CAD build for the part. Positions are in the model's coordinates, mm. Face numbers are marked on the shaded views. A direction names the side the tool comes from. Round coordinates to 2 decimals unless told otherwise and drop trailing zeros. Write each loop counter-clockwise with the first axis right and the second up, starting at its lowest first coordinate (ties: lowest second). Pieces come first, ordered by that corner, then holes. Notation, with made-up numbers: (65, 52.25) - (122, 52.25) arc R24 cw to (122, 62.25) - close; hole circle Ø3 at (35.5, -27.5). An arc over 180 degrees is marked (long way). Answer in a Markdown table with one row per item.
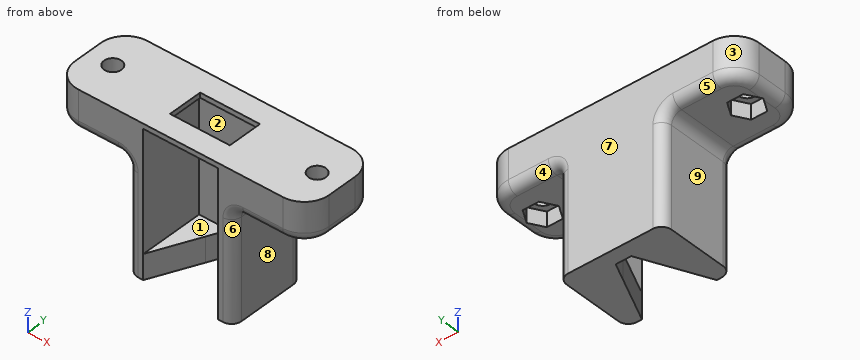
```python
from build123d import *

# Parameters (mm, degrees)
SKETCH1_W           = 15
SKETCH1_H           = 10
SKETCH1_W_2         = 12
SKETCH1_H_2         = 7
SKETCH1_H_3         = 3
SKETCH1_R           = 1.75
BOSS_EXTRUDE1_DEPTH = 1
BOSS_EXTRUDE2_DEPTH = 24
BOSS_EXTRUDE3_START = -7
SKETCH1_5_R         = 1.75
BOSS_EXTRUDE3_DEPTH = 7
BOSS_EXTRUDE4_DEPTH = 5
CUT_EXTRUDE1_DEPTH  = 20
FILLET1_R           = 2


with BuildPart() as part:
    # Sketch1 → Boss-Extrude1 (new body)
    # profile 1 of 7: a face of its own
    with BuildSketch(Plane.XY):
        with Locations((7.5, 5)):
            Rectangle(SKETCH1_W, SKETCH1_H)
        with Locations((7.5, 5)):
            Rectangle(SKETCH1_W_2, SKETCH1_H_2, mode=Mode.SUBTRACT)
    # profile 2 of 7: a face of its own
    with BuildSketch(Plane.XY):
        with Locations((7.5, -1.5)):
            Rectangle(SKETCH1_W, SKETCH1_H_3)
    # profile 3 of 7: a face of its own
    with BuildSketch(Plane.XY):
        Polygon((0, -3), (0, 0), (0, 10), (15, 10), (15, 0), (15, -3), (18, -3), (18, 13), (-3, 13), (-3, -3), align=None)
    # profile 4 of 7: a face of its own
    with BuildSketch(Plane.XY):
        with BuildLine():
            Line((-13, -3), (-3, -3))
            Line((-3, -3), (-3, 13))
            Line((-3, 13), (-13, 13))
            ThreePointArc((-13, 13), (-16.535533906, 11.535533906), (-18, 8))
            Line((-18, 8), (-18, 2))
            ThreePointArc((-18, 2), (-16.535533906, -1.535533906), (-13, -3))
        make_face()
        Polygon((-11.383419246, 7.8), (-9.766838493, 5), (-11.383419246, 2.2), (-14.616580754, 2.2), (-16.233161507, 5), (-14.616580754, 7.8), align=None, mode=Mode.SUBTRACT)
    # profile 5 of 7: a face of its own
    with BuildSketch(Plane.XY):
        Polygon((-14.616580754, 2.2), (-11.383419246, 2.2), (-9.766838493, 5), (-11.383419246, 7.8), (-14.616580754, 7.8), (-16.233161507, 5), align=None)
        with Locations((-13, 5)):
            Circle(SKETCH1_R, mode=Mode.SUBTRACT)
    # profile 6 of 7: a face of its own
    with BuildSketch(Plane.XY):
        with BuildLine():
            Line((18, 13), (18, -3))
            Line((18, -3), (28, -3))
            ThreePointArc((28, -3), (31.535533906, -1.535533906), (33, 2))
            Line((33, 2), (33, 8))
            ThreePointArc((33, 8), (31.535533906, 11.535533906), (28, 13))
            Line((28, 13), (18, 13))
        make_face()
        Polygon((26.383419246, 2.2), (24.766838493, 5), (26.383419246, 7.8), (29.616580754, 7.8), (31.233161507, 5), (29.616580754, 2.2), align=None, mode=Mode.SUBTRACT)
    # profile 7 of 7: a face of its own
    with BuildSketch(Plane.XY):
        Polygon((29.616580754, 7.8), (26.383419246, 7.8), (24.766838493, 5), (26.383419246, 2.2), (29.616580754, 2.2), (31.233161507, 5), align=None)
        with Locations((28, 5)):
            Circle(SKETCH1_R, mode=Mode.SUBTRACT)
    extrude(amount=BOSS_EXTRUDE1_DEPTH)

    # Sketch1<4> → Boss-Extrude2 (add)
    with BuildSketch(Plane.XY):
        Polygon((0, -3), (0, 0), (0, 10), (15, 10), (15, 0), (15, -3), (18, -3), (18, 13), (-3, 13), (-3, -3), align=None)
    extrude(amount=-BOSS_EXTRUDE2_DEPTH)

    # Sketch1<5> → Boss-Extrude3 (add)
    # profile 1 of 4: a face of its own
    with BuildSketch(Plane.XY.offset(BOSS_EXTRUDE3_START)):
        with BuildLine():
            Line((18, 13), (18, -3))
            Line((18, -3), (28, -3))
            ThreePointArc((28, -3), (31.535533906, -1.535533906), (33, 2))
            Line((33, 2), (33, 8))
            ThreePointArc((33, 8), (31.535533906, 11.535533906), (28, 13))
            Line((28, 13), (18, 13))
        make_face()
        Polygon((26.383419246, 2.2), (24.766838493, 5), (26.383419246, 7.8), (29.616580754, 7.8), (31.233161507, 5), (29.616580754, 2.2), align=None, mode=Mode.SUBTRACT)
    # profile 2 of 4: a face of its own
    with BuildSketch(Plane.XY.offset(BOSS_EXTRUDE3_START)):
        Polygon((29.616580754, 7.8), (26.383419246, 7.8), (24.766838493, 5), (26.383419246, 2.2), (29.616580754, 2.2), (31.233161507, 5), align=None)
        with Locations((28, 5)):
            Circle(SKETCH1_5_R, mode=Mode.SUBTRACT)
    # profile 3 of 4: a face of its own
    with BuildSketch(Plane.XY.offset(BOSS_EXTRUDE3_START)):
        with BuildLine():
            Line((-13, -3), (-3, -3))
            Line((-3, -3), (-3, 13))
            Line((-3, 13), (-13, 13))
            ThreePointArc((-13, 13), (-16.535533906, 11.535533906), (-18, 8))
            Line((-18, 8), (-18, 2))
            ThreePointArc((-18, 2), (-16.535533906, -1.535533906), (-13, -3))
        make_face()
        Polygon((-11.383419246, 7.8), (-9.766838493, 5), (-11.383419246, 2.2), (-14.616580754, 2.2), (-16.233161507, 5), (-14.616580754, 7.8), align=None, mode=Mode.SUBTRACT)
    # profile 4 of 4: a face of its own
    with BuildSketch(Plane.XY.offset(BOSS_EXTRUDE3_START)):
        Polygon((-14.616580754, 2.2), (-11.383419246, 2.2), (-9.766838493, 5), (-11.383419246, 7.8), (-14.616580754, 7.8), (-16.233161507, 5), align=None)
        with Locations((-13, 5)):
            Circle(SKETCH1_5_R, mode=Mode.SUBTRACT)
    extrude(amount=BOSS_EXTRUDE3_DEPTH)

    # Sketch2 → Boss-Extrude4 (add)
    with BuildSketch(Plane(origin=(0, 0, -24), x_dir=(-1, 0, 0), z_dir=(0, 0, -1))):
        Polygon((-18, -3), (-15, -3), (-15, 10), (0, 10), (0, -3), (3, -3), (3, 13), (-18, 13), align=None)
        Polygon((-4.316136934, 6.453621675), (0, -3), (0, 10), (-5.935268204, 10), align=None)
        Polygon((-15, 10), (-15, -3), (-10.683863071, 6.453621665), (-9.064731796, 10), align=None)
    extrude(amount=BOSS_EXTRUDE4_DEPTH)

    # Sketch2<4> → Cut-Extrude1 (cut)
    with BuildSketch(Plane(origin=(0, 0, -24), x_dir=(-1, 0, 0), z_dir=(0, 0, -1))):
        Polygon((14.616580754, 7.8), (11.383419246, 7.8), (9.766838493, 5), (11.383419246, 2.2), (14.616580754, 2.2), (16.233161507, 5), align=None)
        Polygon((-29.616580754, 2.2), (-26.383419246, 2.2), (-24.766838493, 5), (-26.383419246, 7.8), (-29.616580754, 7.8), (-31.233161507, 5), align=None)
    extrude(amount=-CUT_EXTRUDE1_DEPTH, mode=Mode.SUBTRACT)

    # Fillet1
    # the kernel refuses this fillet: 2 mm, written as the material it adds along each edge
    with BuildSketch(Plane(origin=(18, 13, -7), x_dir=(1, 0, 0), z_dir=(0, -1, 0)), Plane(origin=(-3, -3, -7), x_dir=(-1, 0, 0), z_dir=(0, 1, 0))) as fillet1_piece_1:
        with BuildLine():
            CenterArc((FILLET1_R, -FILLET1_R), FILLET1_R, 90, 90)
            Line((0, -FILLET1_R), (0, 0))
            Line((0, 0), (FILLET1_R, 0))
        make_face()
    extrude(amount=16)
    # the kernel refuses this fillet: 2 mm, written as the material it takes off along each edge
    with BuildSketch(Plane(origin=(-3, -3, -9), x_dir=(1, 0, 0), z_dir=(0, 0, -1)), Plane(origin=(-3, 13, -34), x_dir=(1, 0, 0), z_dir=(0, 0, 1)), Plane(origin=(18, 13, -9), x_dir=(-1, 0, 0), z_dir=(0, 0, -1)), Plane(origin=(18, -3, -34), x_dir=(-1, 0, 0), z_dir=(0, 0, 1))) as fillet1_2_piece_1:
        with BuildLine():
            CenterArc((FILLET1_R, -FILLET1_R), FILLET1_R, 90, 90)
            Line((0, -FILLET1_R), (0, 0))
            Line((0, 0), (FILLET1_R, 0))
        make_face()
    extrude(amount=25, mode=Mode.SUBTRACT)
    with BuildSketch(Plane(origin=(28, 2, -7), x_dir=(0, -1, 0), z_dir=(-1, 0, 0))) as fillet1_2_piece_2:
        with BuildLine():
            CenterArc((5 - FILLET1_R, FILLET1_R), FILLET1_R, 270, 90)
            Line((5 - FILLET1_R, 0), (5, 0))
            Line((5, 0), (5, FILLET1_R))
        make_face()
    revolve(axis=Axis((28, 2, -7), (0, 0, 1)), revolution_arc=90, mode=Mode.SUBTRACT)
    with BuildSketch(Plane(origin=(20, -3, -7), x_dir=(0, 0, 1), z_dir=(1, 0, 0)), Plane(origin=(28, 13, -7), x_dir=(0, 0, 1), z_dir=(-1, 0, 0)), Plane(origin=(-13, -3, -7), x_dir=(0, 0, 1), z_dir=(1, 0, 0)), Plane(origin=(-5, 13, -7), x_dir=(0, 0, 1), z_dir=(-1, 0, 0))) as fillet1_2_piece_3:
        with BuildLine():
            CenterArc((FILLET1_R, -FILLET1_R), FILLET1_R, 90, 90)
            Line((0, -FILLET1_R), (0, 0))
            Line((0, 0), (FILLET1_R, 0))
        make_face()
    extrude(amount=8, mode=Mode.SUBTRACT)
    with BuildSketch(Plane(origin=(28, 8, -7), x_dir=(1, 0, 0), z_dir=(0, -1, 0))) as fillet1_2_piece_4:
        with BuildLine():
            CenterArc((5 - FILLET1_R, FILLET1_R), FILLET1_R, 270, 90)
            Line((5 - FILLET1_R, 0), (5, 0))
            Line((5, 0), (5, FILLET1_R))
        make_face()
    revolve(axis=Axis((28, 8, -7), (0, 0, 1)), revolution_arc=90, mode=Mode.SUBTRACT)
    with BuildSketch(Plane(origin=(33, 2, -7), x_dir=(0, 0, 1), z_dir=(0, 1, 0)), Plane(origin=(-18, 8, -7), x_dir=(0, 0, 1), z_dir=(0, -1, 0))) as fillet1_2_piece_5:
        with BuildLine():
            CenterArc((FILLET1_R, -FILLET1_R), FILLET1_R, 90, 90)
            Line((0, -FILLET1_R), (0, 0))
            Line((0, 0), (FILLET1_R, 0))
        make_face()
    extrude(amount=6, mode=Mode.SUBTRACT)
    with BuildSketch(Plane(origin=(-13, 2, -7), x_dir=(-1, 0, 0), z_dir=(0, 1, 0))) as fillet1_2_piece_6:
        with BuildLine():
            CenterArc((5 - FILLET1_R, FILLET1_R), FILLET1_R, 270, 90)
            Line((5 - FILLET1_R, 0), (5, 0))
            Line((5, 0), (5, FILLET1_R))
        make_face()
    revolve(axis=Axis((-13, 2, -7), (0, 0, 1)), revolution_arc=90, mode=Mode.SUBTRACT)
    with BuildSketch(Plane(origin=(-13, 8, -7), x_dir=(0, 1, 0), z_dir=(1, 0, 0))) as fillet1_2_piece_7:
        with BuildLine():
            CenterArc((5 - FILLET1_R, FILLET1_R), FILLET1_R, 270, 90)
            Line((5 - FILLET1_R, 0), (5, 0))
            Line((5, 0), (5, FILLET1_R))
        make_face()
    revolve(axis=Axis((-13, 8, -7), (0, 0, 1)), revolution_arc=90, mode=Mode.SUBTRACT)
    with BuildSketch(Plane(origin=(-5, 13, -9), x_dir=(0, 0, 1), z_dir=(-1, 0, 0))) as fillet1_2_piece_8:
        with BuildLine():
            CenterArc((2 + FILLET1_R, -FILLET1_R), FILLET1_R, 90, 90)
            Line((2, -FILLET1_R), (2, 0))
            Line((2, 0), (2 + FILLET1_R, 0))
        make_face()
    revolve(axis=Axis((-5, 13, -9), (0, 1, 0)), revolution_arc=90, mode=Mode.SUBTRACT)
    with BuildSketch(Plane(origin=(-5, -3, -9), x_dir=(0, 0, 1), z_dir=(-1, 0, 0))) as fillet1_2_piece_9:
        with BuildLine():
            CenterArc((2 + FILLET1_R, FILLET1_R), FILLET1_R, 180, 90)
            Line((2, FILLET1_R), (2, 0))
            Line((2, 0), (2 + FILLET1_R, 0))
        make_face()
    revolve(axis=Axis((-5, -3, -9), (0, 1, 0)), revolution_arc=90, mode=Mode.SUBTRACT)
    with BuildSketch(Plane(origin=(20, 13, -9), x_dir=(0, 0, 1), z_dir=(1, 0, 0))) as fillet1_2_piece_10:
        with BuildLine():
            CenterArc((2 + FILLET1_R, FILLET1_R), FILLET1_R, 180, 90)
            Line((2, FILLET1_R), (2, 0))
            Line((2, 0), (2 + FILLET1_R, 0))
        make_face()
    revolve(axis=Axis((20, 13, -9), (0, -1, 0)), revolution_arc=90, mode=Mode.SUBTRACT)
    with BuildSketch(Plane(origin=(20, -3, -9), x_dir=(0, 0, 1), z_dir=(1, 0, 0))) as fillet1_2_piece_11:
        with BuildLine():
            CenterArc((2 + FILLET1_R, -FILLET1_R), FILLET1_R, 90, 90)
            Line((2, -FILLET1_R), (2, 0))
            Line((2, 0), (2 + FILLET1_R, 0))
        make_face()
    revolve(axis=Axis((20, -3, -9), (0, -1, 0)), revolution_arc=90, mode=Mode.SUBTRACT)


solid = part.part
```
Q1. Saw through at B-B on z = -25. List the corners of the cut face in (x, y), then the cut area to 3 significant figures.
Computed:
| item | result |
|---|---|
| outline | (-3, -1) arc R2 ccw to (-1, -3) - (0, -3) - (5.94, 10) - (9.06, 10) - (15, -3) - (16, -3) arc R2 ccw to (18, -1) - (18, 11) arc R2 ccw to (16, 13) - (-1, 13) arc R2 ccw to (-3, 11) - close |
| area | 215 mm2 |
Q2. Saw through at A-A on z = -2. List the corners of the cut face in (x, y), then the cut area to 3 significant figures.
Computed:
| item | result |
|---|---|
| outline | (-18, 2) arc R5 ccw to (-13, -3) - (0, -3) - (0, 10) - (15, 10) - (15, -3) - (28, -3) arc R5 ccw to (33, 2) - (33, 8) arc R5 ccw to (28, 13) - (-13, 13) arc R5 ccw to (-18, 8) - close; hole circle Ø3.5 at (-13, 5); hole circle Ø3.5 at (28, 5) |
| area | 580 mm2 |
Q3. Saw through at C-C on x = 11.5. List the corners of the cut face in (y, z), then the cut area to 3 significant figures.
Computed:
| item | result |
|---|---|
| outline | (-3, 0) - (1.5, 0) - (1.5, 1) - (-3, 1) - close; (4.67, -29) - (13, -29) - (13, 1) - (8.5, 1) - (8.5, 0) - (10, 0) - (10, -24) - (4.67, -24) - close |
| area | 123 mm2 |
Q4. Saw through at D-D on z = -19.75. List the corners of the cut face in (x, y).
Computed:
| item | result |
|---|---|
| outline | (-3, -1) arc R2 ccw to (-1, -3) - (0, -3) - (0, 10) - (15, 10) - (15, -3) - (16, -3) arc R2 ccw to (18, -1) - (18, 11) arc R2 ccw to (16, 13) - (-1, 13) arc R2 ccw to (-3, 11) - close |
Q5. Drill centre lines: line 1 (X direction, y = 5, z = -1.5); line 2 (X direction, y = -0.5, z = -20.75); line 3 (Z direction, x = 20.5, y = 2.25). Where is each one in solid material? Low to high.
Computed:
| item | result |
|---|---|
| line 1 | x = -18 to -14.75, -11.25 to 0, 15 to 26.25, 29.75 to 33 |
| line 2 | x = -3 to 0, 15 to 18 |
| line 3 | z = -7 to 1 |
Q6. Pull direction Z, two halves, no side cores. Call the marked faces 1, 2, 3 and 4: released by +Z, released by -Z, zero draft, split by the parting line, or undercut.
Computed:
| item | result |
|---|---|
| face 1 | undercut |
| face 2 | undercut |
| face 3 | zero draft |
| face 4 | released by -Z |
Q7. Flat gauge pins, fed straight in: pin 1 (3 mm diameter, centred on y = 3, z = -26, fed in from -X); pin 2 (3 mm diameter, centred on x = 26.5, y = 4.5, fed in from -Z); pin 3 (6.5 mm diameter, centred on y = 5.5, z = -10.5, fed in from -X). Where does each tip first touch, or does it go through?
Computed:
| item | result |
|---|---|
| pin 1 | stops at x = -3 |
| pin 2 | stops at z = -7 |
| pin 3 | stops at x = -4.03 |
Q8. 3-axis set-ups, long thin cutter, end or side, ignore diameter. For the marked faces 5, 6, 7, 8 and 9: which of +Z, -Z, +X, -X, +Y, -Y reach the whole face in a straight line?
Computed:
| item | result |
|---|---|
| face 5 | -Z, -X, +Y |
| face 6 | -Z, +X, -Y |
| face 7 | +Z, -Z, +X, -X, +Y |
| face 8 | -Z, +X, +Y, -Y |
| face 9 | -Z, -X, +Y, -Y |
